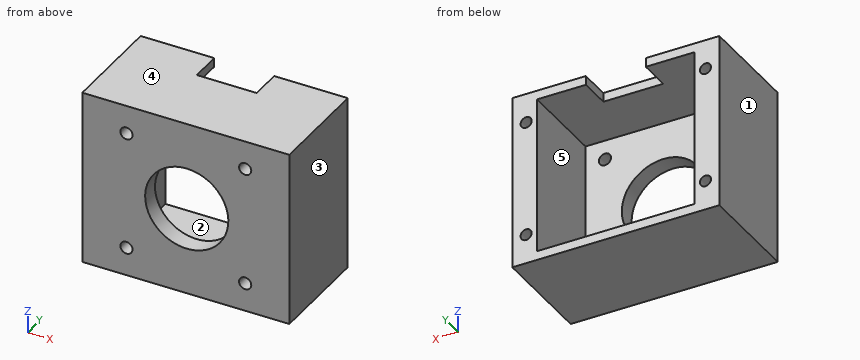
Autodesk Inventor part; units mm, degrees
ref_plane "YZ Plane" through (0, 0, 0) normal (1, 0, 0) x (0, 1, 0)
ref_plane "XZ Plane" through (0, 0, 0) normal (0, 1, 0) x (-1, 0, 0)
ref_plane "XY Plane" through (0, 0, 0) normal (0, 0, 1) x (1, 0, 0)
sketch "スケッチ1" plane through (0, 0, 0) normal (0, 1, 0) x (-1, 0, 0)
  line L0 (0, 0) -> (-56, 0)
  line L1 (-56, 0) -> (-56, -47.5)
  line L2 (-56, -47.5) -> (0, -47.5)
  line L3 (0, -47.5) -> (0, 0)
  line L4 (-7.5, -3) -> (-49, -3)
  line L5 (-49, -3) -> (-49, -44.5)
  line L6 (-49, -44.5) -> (-7.5, -44.5)
  line L7 (-7.5, -44.5) -> (-7.5, -3)
  dimension "d0" = 56
  dimension "d1" = 47.5
  dimension "d6" = 41.5
  dimension "d7" = 41.5
extrude "押し出し1" add sketch "スケッチ1" along normal blind 28.4 contours L3 L2 L1 L0 | L7 L6 L5 L4
ref_plane "作業平面2" through (0, 28.4, 0) normal (0, 1, 0) x (1, 0, 0)
sketch "スケッチ3" plane through (0, 28.4, 0) normal (0, 1, 0) x (1, 0, 0)
  line L0 (6.7, 2.45) -> (49.3, 2.45)
  line L1 (49.3, 2.45) -> (49.3, 45.05)
  line L2 (49.3, 45.05) -> (6.7, 45.05)
  line L3 (6.7, 45.05) -> (6.7, 2.45)
  line L4 (56, 47.5) -> (0, 47.5)
  line L5 (0, 0) -> (56, 0)
  line L6 (56, 0) -> (56, 47.5)
  point P0 (28, 45.05)
  point P1 (28, 47.5)
  point P2 (28, 0)
  point P3 (49.3, 23.75)
  point P4 (56, 23.75)
  point P5 (56, 23.75)
  dimension "d8" = 42.6
  dimension "d9" = 42.6
  dimension "d61" = 0
  dimension "d62" = 0
extrude "押し出し2" cut sketch "スケッチ3" against normal blind 23.6
sketch "スケッチ4" plane through (0, 4.8, 0) normal (0, 1, 0) x (1, 0, 0)
  line L0 (6.7, 2.45) -> (6.7, 45.05)
  line L1 (49.3, 45.05) -> (49.3, 2.45)
  line L2 (6.7, 45.05) -> (49.3, 45.05)
  point P0 (0, 0)
  point P1 (28.25, 23.75)
hole "穴1" at (28.25, 4.8, -23.75) direction (0, -1, 0) diameter 22.5 end through all
sketch "スケッチ5" plane through (0, 4.8, 0) normal (0, 1, 0) x (1, 0, 0)
  line L0 (6.7, 45.05) -> (49.3, 45.05)
  line L1 (6.7, 2.45) -> (6.7, 45.05)
  line L2 (49.3, 45.05) -> (49.3, 2.45)
  line L3 (49.3, 2.45) -> (6.7, 2.45)
  point P0 (0, 0)
  point P1 (11.95, 39.8)
  point P2 (44.05, 39.8)
  point P3 (44.05, 7.7)
  point P4 (11.95, 7.7)
  dimension "d23" = 5.25
  dimension "d24" = 5.25
  dimension "d25" = 5.25
  dimension "d26" = 5.25
  dimension "d27" = 5.25
  dimension "d28" = 5.25
  dimension "d29" = 5.25
  dimension "d30" = 5.25
hole "穴2" at (11.95, 4.8, -39.8) at (44.05, 4.8, -39.8) at (44.05, 4.8, -7.7) at (11.95, 4.8, -7.7) direction (0, -1, 0) diameter 3.3 end through all
sketch "スケッチ6" plane through (0, 28.4, 0) normal (0, 1, 0) x (1, 0, 0)
  line L0 (0, 47.5) -> (0, 0)
  line L1 (49.3, 45.05) -> (49.3, 2.45)
  line L2 (56, 47.5) -> (0, 47.5)
  line L3 (0, 0) -> (56, 0)
  line L4 (56, 0) -> (56, 47.5)
  line L5 (6.7, 2.45) -> (6.7, 45.05)
  point P0 (3.75, 39.5)
  point P1 (3.75, 8)
  point P2 (52.25, 8)
  point P3 (52.25, 39.5)
  dimension "d38" = 3.75
  dimension "d40" = 8
  dimension "d41" = 8
  dimension "d42" = 3.75
  dimension "d43" = 3.75
  dimension "d44" = 8
  dimension "d45" = 8
  dimension "d46" = 3.75
  dimension "d64" = 2.95
hole "穴3" at (3.75, 28.4, -39.5) at (3.75, 28.4, -8) at (52.25, 28.4, -8) at (52.25, 28.4, -39.5) direction (0, -1, 0) diameter 3 depth 15
sketch "スケッチ7" plane through (0, 0, 0) normal (0, 0, 1) x (1, 0, 0)
  line L0 (56, 28.4) -> (0, 28.4)
  line L1 (19.9, 28.4) -> (36.1, 28.4)
  line L2 (36.1, 28.4) -> (36.1, 19.9)
  line L3 (36.1, 19.9) -> (19.9, 19.9)
  line L4 (19.9, 19.9) -> (19.9, 28.4)
  line L5 (0, 0) -> (56, 0)
  point P0 (28, 19.9)
  point P1 (28, 0)
  dimension "d55" = 16.2
  dimension "d63" = 0
extrude "押し出し3" cut sketch "スケッチ7" against normal blind 3
properties part number "motor_case2_3D プリント"
Here's how the part is built. I have some questions about the finished solid (model axes, mm). Face numbers are marked on the shaded views. A direction names the side the tool comes from. Coordinates: 2 decimals unless noted, no trailing zeros. Write each loop counter-clockwise with the first axis right and the second up, starting at its lowest first coordinate (ties: lowest second). Pieces come first, ordered by that corner, then holes.
1) Thinking about a two-plate mould opening in Z: for the marked faces 3, 4 and 5, which applies, +Z half, -Z half, draft (parallel to the pull), parting line (faces both ways), or undercut?
Filled in:
face 3: draft
face 4: +Z half
face 5: undercut
2) If we section it at D-D (y = 15.5): List the corners of the cut face in (x, z) for me.
Filled in:
outline: (0, -47.5) - (56, -47.5) - (56, 0) - (0, 0) - close; hole circle Ø3 at (3.75, -39.5); hole circle Ø3 at (3.75, -8); hole (6.7, -45.05) - (49.3, -45.05) - (49.3, -2.45) - (6.7, -2.45) - close; hole circle Ø3 at (52.25, -39.5); hole circle Ø3 at (52.25, -8)
3) Which directions (+Z, -Z, +X, -X, +Y, -Y) give clear straight access to the entire face, cutting with the end or side of a thin tool? Please do the marked faces 1 and 2.
Filled in:
face 1: +Z, -Z, -X, +Y, -Y
face 2: +Y
4) I'm going to push flat-ended pins straight in: pin 1 (1 mm diameter, centred on x = 8, z = -19.5, fed in from +Y); pin 2 (1.5 mm diameter, centred on x = 4, z = -8, fed in from +Y); pin 3 (2.5 mm diameter, centred on x = 26.5, z = -1, fed in from +Y). Where does each tip first touch, or does it pass through?
Filled in:
pin 1: stops at y = 4.8
pin 2: stops at y = 13.4
pin 3: stops at y = 19.9
5) If we section it at A-A (z = -23.75): List the corners of the cut face in (x, y) for me.
Filled in:
outline: (0, 0) - (17, 0) - (17, 4.8) - (6.7, 4.8) - (6.7, 28.4) - (0, 28.4) - close; (39.5, 0) - (56, 0) - (56, 28.4) - (49.3, 28.4) - (49.3, 4.8) - (39.5, 4.8) - close
6) If I drill on line 1 (Z direction, x = 52.25, y = 17.75); line 2 (Z direction, x = 11.95, y = 3.45); line 3 (X direction, y = 17.75, z = -8), over which ranges is the centre line in solid material (lowest first)?
Filled in:
line 1: z = -47.5 to -41, -38 to -9.5, -6.5 to 0
line 2: z = -47.5 to -41.45, -38.15 to -9.35, -6.05 to 0
line 3: x = 0 to 2.25, 5.25 to 6.7, 49.3 to 50.75, 53.75 to 56
7) If we section it at C-C (y = 5.75): List the corners of the cut face in (x, z) for me.
Filled in:
outline: (0, -47.5) - (56, -47.5) - (56, 0) - (0, 0) - close; hole (6.7, -45.05) - (49.3, -45.05) - (49.3, -2.45) - (6.7, -2.45) - close
8) If we section it at B-B (x = 28.25): List the corners of the cut face in (y, z) for me, plus the area to 3 significant figures.
Filled in:
outline: (0, -47.5) - (28.4, -47.5) - (28.4, -45.05) - (4.8, -45.05) - (4.8, -35) - (0, -35) - close; (0, -12.5) - (4.8, -12.5) - (4.8, -2.45) - (19.9, -2.45) - (19.9, 0) - (0, 0) - close
area: 215 mm2
